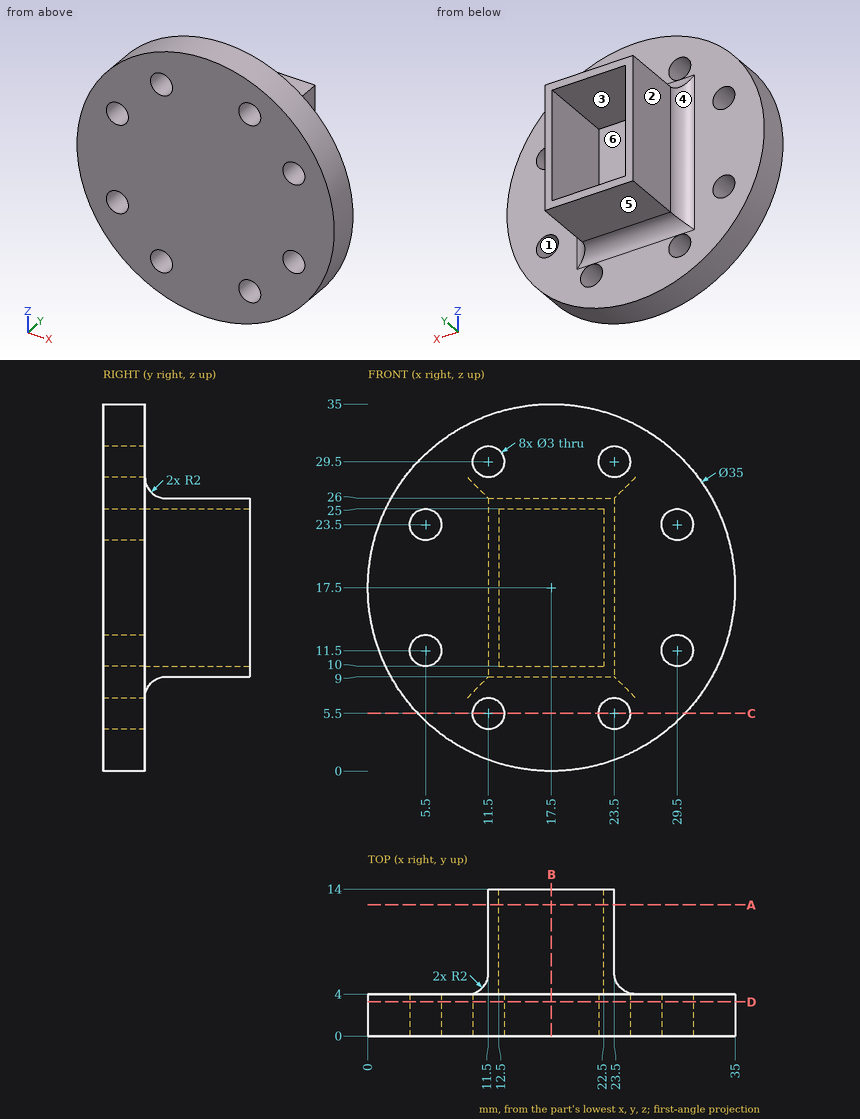
Study the drawing (mm; zero at the part's minimum x, y, z) and answer. A direction names the side the tool comes from. Coordinates: 2 decimals unless noted, no trailing zeros. Loops run counter-clockwise (first coordinate to the right, second up) from the corner with the lowest first, then second, coordinate; pieces in that order, holes last. Notation, with made-up numbers: (-35.5, 28.5) -> (17.5, 28.5) arc R27 cw to (17.5, 66.5) -> close; hole circle Ø8 at (-38.5, 3.5). An arc over 180 degrees is marked (long way). Answer as CSV lines item,"result".
1) The part is cut by section C-C (z = 5.5). Give the vertices of the cut face in (x, y), and give its area (3 significant figures).
A:
outline,"(4.76, 0) -> (10, 0) -> (10, 4) -> (4.76, 4) -> close; (13, 0) -> (22, 0) -> (22, 4) -> (13, 4) -> close; (25, 0) -> (30.24, 0) -> (30.24, 4) -> (25, 4) -> close"
area,"77.9 mm²"
2) For a pull along Z with two mould halves and no side action, classify the marked faces 4, 5 and 6 as released by +Z, released by -Z, zero draft, split by the parting line, or undercut.
A:
face 4,"zero draft"
face 5,"released by -Z"
face 6,"undercut"
3) For the marked faces 1, 2 and 3, determine the directions among +Z, -Z, +X, -X, +Y, -Y from which every point of the face is accessible in a straight line to the end or side of a thin tool.
A:
face 1,"+Y, -Y"
face 2,"+Z, -Z, -X, +Y"
face 3,"+Y"
4) Flat-ended cylindrical pins translate along their axes: pin 1 (5 mm diameter, centred on x = 21.5, y = 10.5, fed in from -Z); pin 2 (2.5 mm diameter, centred on y = 11.5, z = 19.5, fed in from -X); pin 3 (5 mm diameter, centred on x = 29.5, y = 2.5, fed in from -Z); pin 4 (4 mm diameter, centred on x = 16, y = 2.5, fed in from +Z). Find the tip coordinate at first contact, or state that the pin passes through.
A:
pin 1,"stops at z = 9"
pin 2,"stops at x = 11.5"
pin 3,"stops at z = 2.8"
pin 4,"stops at z = 35"
5) Straight lines are drawn through the part: probe 1 along Z at (x, y) = (15.5, 11.5); probe 2 along X at (y, z) = (9.5, 16.5); probe 3 along X at (y, z) = (3.15, 5.5). For each, find the intervals that lie inside material, in ascending order.
A:
probe 1,"z = 9 to 10, 25 to 26"
probe 2,"x = 11.5 to 12.5, 22.5 to 23.5"
probe 3,"x = 4.76 to 10, 13 to 22, 25 to 30.24"
6) The part is cut by section B-B (x = 17.5). Give the vertices of the cut face in (y, z).
A:
outline,"(0, 0) -> (4, 0) -> (4, 7) arc R2 cw to (6, 9) -> (14, 9) -> (14, 10) -> (4, 10) -> (4, 25) -> (14, 25) -> (14, 26) -> (6, 26) arc R2 cw to (4, 28) -> (4, 35) -> (0, 35) -> close"
7) The part is cut by section D-D (y = 3.25). State how many separate pieces and enclosed holes the cut face has, and give its area (3 significant figures).
A:
separate pieces,"1"
enclosed holes,"8"
area,"906 mm²"
8) The part is cut by section A-A (y = 12.5). Give the vertices of the cut face in (x, z).
A:
outline,"(11.5, 9) -> (23.5, 9) -> (23.5, 26) -> (11.5, 26) -> close; hole (12.5, 10) -> (22.5, 10) -> (22.5, 25) -> (12.5, 25) -> close"
